Part print with two shaded views. Sizes in mm from the minimum x, y, z corner. A direction names the side the tool comes from. Round coordinates to 2 decimals unless told otherwise and drop trailing zeros. Write each loop counter-clockwise with the first axis right and the second up, starting at its lowest first coordinate (ties: lowest second). Pieces come first, ordered by that corner, then holes. Notation, with made-up numbers: (10, 61.5) -> (25, 61.5) arc R24 cw to (25, 71.5) -> close; hole circle Ø9 at (5.5, -18). An arc over 180 degrees is marked (long way). Answer in a Markdown table with one row per item. Add a question column.
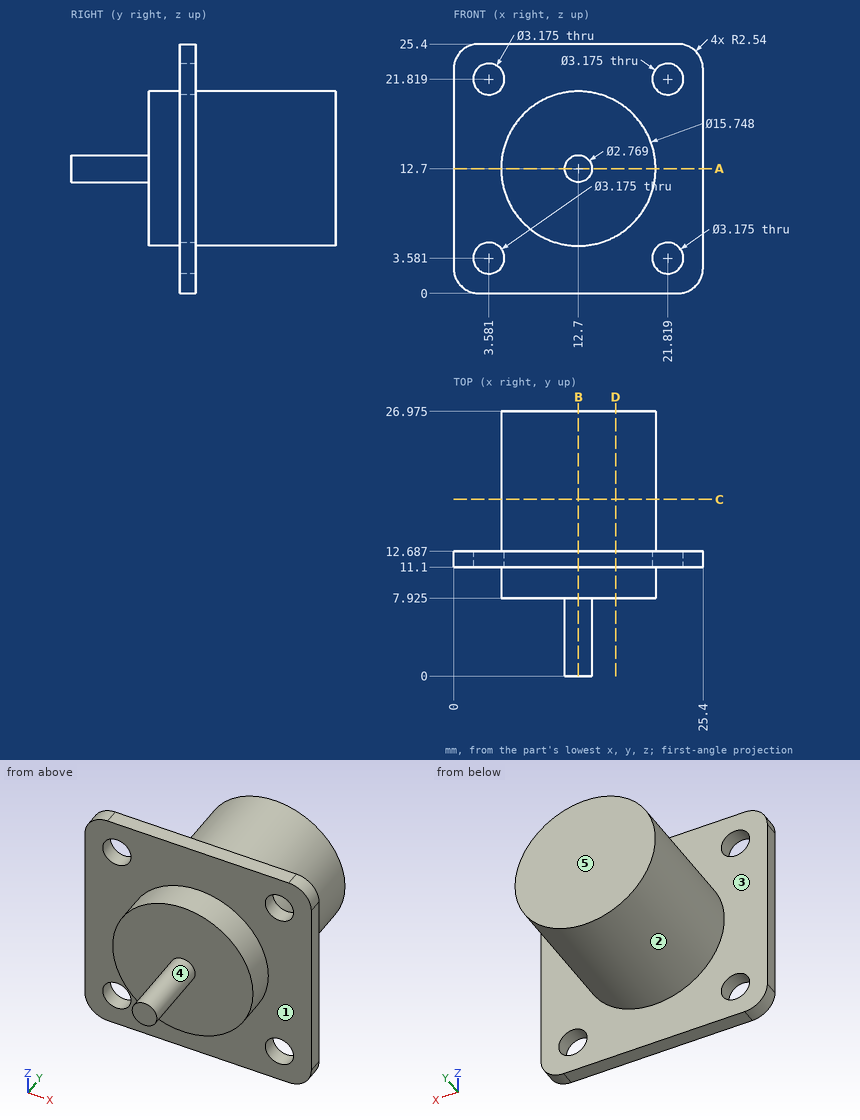
Item 1: Pin check, flat tips, straight feed: pin 1 (5 mm diameter, centred on x = 3.58, z = 3.58, fed in from +Y); pin 2 (5 mm diameter, centred on y = 4.5, z = 3, fed in from +X); pin 3 (6 mm diameter, centred on x = 13.5, y = 19.5, fed in from +Z); pin 4 (2 mm diameter, centred on y = 20, z = 9, fed in from -X). Stop position of each tip, or through.
Item 2: Drill centre lines: probe 1 along Y at (x, z) = (18, 9) (1 decimal); probe 2 along Y at (x, z) = (1, 23.25); probe 3 along X at (y, z) = (12.75, 17) (1 decimal). Where is each one in solid material? Low to high.
Item 3: Two-plate mould, pull along Z, no slides. Class the marked faces 1 and 2: +Z half, -Z half, draft (parallel to the pull), parting line (faces both ways), or undercut.
Item 4: Saw through at D-D on x = 16.5. Give the cut face in (y, z) (1 decimal), then the cut area to 3 significant figures.
Item 5: Tool access for the marked faces 3, 4 and 5: list every direction of +Z, -Z, +X, -X, +Y, -Y with a clear straight run to the whole face (end or side of a thin tool).
Item 6: Saw through at A-A on z = 12.7. Give the cut face in (x, y) (1 decimal).
Item 7: Saw through at C-C on y = 18. Give the cut face in (x, z).
Item 8: Saw through at B-B on x = 12.7. Give the cut face in (y, z) (1 decimal).
Recorded:
| question | item | result |
|---|---|---|
| 1 | pin 1 | y = 12.69 |
| 1 | pin 2 | through |
| 1 | pin 3 | z = 20.57 |
| 1 | pin 4 | x = 5.3 |
| 2 | probe 1 | 7.9 to 27 |
| 2 | probe 2 | 11.1 to 12.69 |
| 2 | probe 3 | 6.1 to 19.3 |
| 3 | face 1 | draft |
| 3 | face 2 | parting line |
| 4 | outline | (7.9, 5.8) -> (11.1, 5.8) -> (11.1, 0) -> (12.7, 0) -> (12.7, 5.8) -> (27, 5.8) -> (27, 19.6) -> (12.7, 19.6) -> (12.7, 25.4) -> (11.1, 25.4) -> (11.1, 19.6) -> (7.9, 19.6) -> close |
| 4 | area | 281 mm2 |
| 5 | face 3 | +Y |
| 5 | face 4 | -Y |
| 5 | face 5 | +Z, -Z, +X, -X, +Y |
| 6 | outline | (0, 11.1) -> (4.8, 11.1) -> (4.8, 7.9) -> (11.3, 7.9) -> (11.3, 0) -> (14.1, 0) -> (14.1, 7.9) -> (20.6, 7.9) -> (20.6, 11.1) -> (25.4, 11.1) -> (25.4, 12.7) -> (20.6, 12.7) -> (20.6, 27) -> (4.8, 27) -> (4.8, 12.7) -> (0, 12.7) -> close |
| 7 | outline | circle Ø15.75 at (12.7, 12.7) |
| 8 | outline | (0, 11.3) -> (7.9, 11.3) -> (7.9, 4.8) -> (11.1, 4.8) -> (11.1, 0) -> (12.7, 0) -> (12.7, 4.8) -> (27, 4.8) -> (27, 20.6) -> (12.7, 20.6) -> (12.7, 25.4) -> (11.1, 25.4) -> (11.1, 20.6) -> (7.9, 20.6) -> (7.9, 14.1) -> (0, 14.1) -> close |
